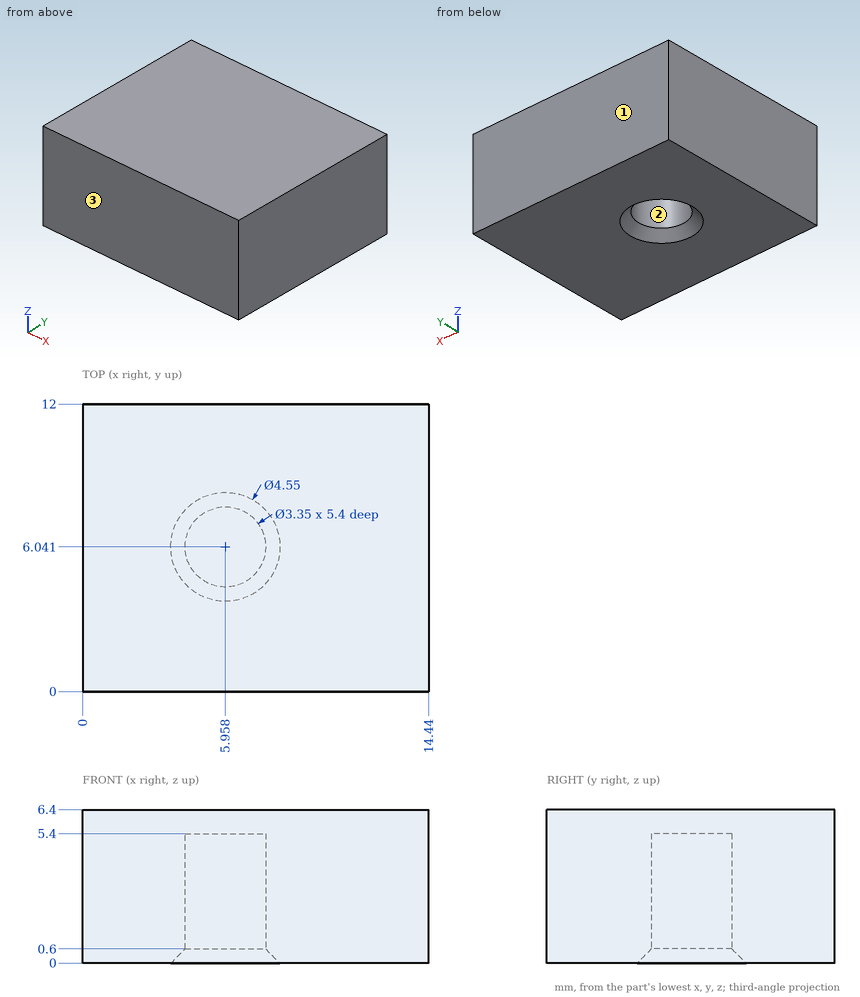
Here's the drawing with two shaded views (mm, measured from the low corner). I have some questions. Coordinates: 2 decimals unless noted, no trailing zeros. Put each result on its own line as item: value. Start each with the question number.
(1) I need wall thicknesses on probe 1 along X at (y, z) = (5, 1.25) (1 decimal); probe 2 along Y at (x, z) = (5.25, 3.75) (1 decimal); probe 3 along Y at (x, z) = (5, 4.5) (1 decimal). Which ranges of each line are inside material? Lowest first, please.
(2) Will this pin go through, and if not, where does the flat tip stop? pin 1 Ø1 at (x, y) = (6.5, 6) entering from -Z.
(3) We'd pull the mould along Y, two halves only. Please class the marked faces 1, 2 and 3: +Y half, -Y half, draft (parallel to the pull), parting line (faces both ways), or undercut.
Worked answers:
1. probe 1: x = 0 to 4.6, 7.3 to 14.4
1. probe 2: y = 0 to 4.5, 7.6 to 12
1. probe 3: y = 0 to 4.7, 7.4 to 12
2. pin 1: stops at z = 5.4
3. face 1: +Y half
3. face 2: undercut
3. face 3: -Y half
